For this review, take the finished solid that the model builds, in its own axes (mm). A direction names the side the tool comes from. Coordinates: 2 decimals unless noted, no trailing zeros. Loops run counter-clockwise (first coordinate to the right, second up) from the corner with the lowest first, then second, coordinate; pieces in that order, holes last. Notation, with made-up numbers: (-25.75, 40) -> (6.25, 40) arc R14 cw to (6.25, 61) -> close; hole circle Ø1 at (-10.5, 32). An arc over 180 degrees is marked (long way). One line per item, written item: value.
from build123d import *

# Parameters (mm, degrees)
SKETCH_1_W              = 200
SKETCH_1_H              = 213
EXTRUDE_1_DEPTH         = 4
EXTRUDE_2_DEPTH         = 54
CUT_EXTRUDE_2_DEPTH     = 298.880848663
CUT_EXTRUDE_3_DEPTH     = 42
SKETCH_7_R              = 1.8
SKETCH_7_R_2            = 11.5
CUT_EXTRUDE_4_DEPTH     = 282.53330176
MIRROR_START            = 176
MIRROR_1_OUTLINE_R      = 1.8
MIRROR_1_OUTLINE_R_2    = 11.5
MIRROR_1_DEPTH          = 3.5
CUT_EXTRUDE_START       = -21
CUT_EXTRUDE_5_OUTLINE_W = 27
CUT_EXTRUDE_5_OUTLINE_H = 20
CUT_EXTRUDE_5_DEPTH     = 21
CUT_EXTRUDE_START_2     = -6
CUT_EXTRUDE_6_OUTLINE_W = 27
CUT_EXTRUDE_6_OUTLINE_H = 28
CUT_EXTRUDE_6_DEPTH     = 6
CHAMFER_1_SIZE          = 4
CUT_EXTRUDE_START_3     = -54
CUT_EXTRUDE_7_DEPTH     = 54
EXTRUDE_3_DEPTH         = 10


# Read off the part's stored shape, not the designer's step: 镜向1, 切除-拉伸5, 切除-拉伸6
with BuildPart() as part:
    # 草图1 → 凸台-拉伸1 (new body)
    with BuildSketch(Plane(origin=(0, 0, 0), x_dir=(1, 0, 0), z_dir=(0, 1, 0))):
        with Locations((100, 106.5)):
            Rectangle(SKETCH_1_W, SKETCH_1_H)
    extrude(amount=EXTRUDE_1_DEPTH)

    # 草图1<4> → 凸台-拉伸2 (add)
    with BuildSketch(Plane(origin=(0, 0, 0), x_dir=(1, 0, 0), z_dir=(0, 1, 0))):
        with BuildLine():
            Line((0, 213), (0, 0))
            ThreePointArc((0, 0), (21.966991411, 53.033008589), (75, 75))
            Line((75, 75), (75, 213))
            Line((75, 213), (0, 213))
        make_face()
        with BuildLine():
            Line((125, 213), (125, 75))
            ThreePointArc((125, 75), (178.033008589, 53.033008589), (200, 0))
            Line((200, 0), (200, 213))
            Line((200, 213), (125, 213))
        make_face()
    extrude(amount=-EXTRUDE_2_DEPTH)

    # 草图3 → 切除-拉伸2 (cut, through all)
    with BuildSketch(Plane.XZ.offset(54)):
        Polygon((20.5, -186), (20.5, -165), (20.5, -144), (20.5, -117), (0, -117), (0, -213), (20.5, -213), align=None)
        Polygon((179.5, -117), (200, -117), (200, -213), (179.5, -213), (179.5, -165), align=None)
    extrude(amount=-CUT_EXTRUDE_2_DEPTH, mode=Mode.SUBTRACT)

    # 草图5 → 切除-拉伸3 (cut)
    with BuildSketch(Plane.XZ.offset(54)):
        Polygon((176, -165), (176, -144), (125, -144), (125, -186), (176, -186), align=None)
        Polygon((24, -165), (24, -144), (75, -144), (75, -186), (24, -186), align=None)
    extrude(amount=-CUT_EXTRUDE_3_DEPTH, mode=Mode.SUBTRACT)

    # 草图7 → 切除-拉伸4 (cut, through all)
    with BuildSketch(Plane(origin=(24, 0, 0), x_dir=(0, 0, -1), z_dir=(1, 0, 0))):
        with Locations((180.5, -17.5)):
            Circle(SKETCH_7_R)
        with Locations((149.5, -17.5)):
            Circle(SKETCH_7_R)
        with Locations((165, -33)):
            Circle(SKETCH_7_R_2)
        with Locations((180.5, -48.5)):
            Circle(SKETCH_7_R)
        with Locations((149.5, -48.5)):
            Circle(SKETCH_7_R)
    extrude(amount=-CUT_EXTRUDE_4_DEPTH, mode=Mode.SUBTRACT)

    # 镜向1 outline → 镜向1 (cut)
    with BuildSketch(Plane.YZ.offset(MIRROR_START)):
        with Locations((-17.5, -180.5)):
            Circle(MIRROR_1_OUTLINE_R)
        with Locations((-17.5, -149.5)):
            Circle(MIRROR_1_OUTLINE_R)
        with Locations((-33, -165)):
            Circle(MIRROR_1_OUTLINE_R_2)
        with Locations((-48.5, -180.5)):
            Circle(MIRROR_1_OUTLINE_R)
        with Locations((-48.5, -149.5)):
            Circle(MIRROR_1_OUTLINE_R)
    extrude(amount=MIRROR_1_DEPTH, mode=Mode.SUBTRACT)

    # 切除-拉伸5 outline → 切除-拉伸5 (cut)
    with BuildSketch(Plane(origin=(75, 0, 0), x_dir=(0, 0, -1), z_dir=(1, 0, 0)).offset(CUT_EXTRUDE_START)):
        with Locations((199.5, -33)):
            Rectangle(CUT_EXTRUDE_5_OUTLINE_W, CUT_EXTRUDE_5_OUTLINE_H)
    extrude(amount=CUT_EXTRUDE_5_DEPTH, mode=Mode.SUBTRACT)

    # 切除-拉伸6 outline → 切除-拉伸6 (cut)
    with BuildSketch(Plane.ZY.offset(-125).offset(CUT_EXTRUDE_START_2)):
        with Locations((-199.5, -33)):
            Rectangle(CUT_EXTRUDE_6_OUTLINE_W, CUT_EXTRUDE_6_OUTLINE_H)
    extrude(amount=CUT_EXTRUDE_6_DEPTH, mode=Mode.SUBTRACT)

    # 倒角1
    chamfer_1_edges = [part.edges().sort_by_distance(p)[0] for p in [
        (20.5, -25, -117),
        (179.5, -25, -117),
    ]]
    chamfer(chamfer_1_edges, length=CHAMFER_1_SIZE)

    # 草图11 → 切除-拉伸7 (cut)
    with BuildSketch(Plane.XZ.offset(54).offset(CUT_EXTRUDE_START_3)):
        with BuildLine():
            Line((75, -144), (10.975621098, -39.0625))
            ThreePointArc((10.975621098, -39.0625), (38.289562111, -65.401404801), (75, -75))
            Line((75, -75), (75, -144))
        make_face()
        with BuildLine():
            Line((125, -144), (125, -75))
            ThreePointArc((125, -75), (161.710437889, -65.401404801), (189.024378902, -39.0625))
            Line((189.024378902, -39.0625), (125, -144))
        make_face()
    extrude(amount=CUT_EXTRUDE_7_DEPTH, mode=Mode.SUBTRACT)

    # 草图12 → 凸台-拉伸3 (add)
    with BuildSketch(Plane(origin=(0, -54, 0), x_dir=(-1, 0, 0), z_dir=(0, -1, 0))):
        with BuildLine():
            Line((-9.993972793, 71.605361452), (-1.667158175, 86.766701767))
            ThreePointArc((-1.667158175, 86.766701767), (0, 93.265459675), (-1.667158175, 99.764217583))
            Line((-1.667158175, 99.764217583), (-9.993972793, 114.925557899))
            ThreePointArc((-9.993972793, 114.925557899), (-13.5, 117), (-17.006027207, 114.925557899))
            Line((-17.006027207, 114.925557899), (-25.332841825, 99.764217583))
            ThreePointArc((-25.332841825, 99.764217583), (-27, 93.265459675), (-25.332841825, 86.766701767))
            Line((-25.332841825, 86.766701767), (-17.006027207, 71.605361452))
            ThreePointArc((-17.006027207, 71.605361452), (-13.5, 69.53091935), (-9.993972793, 71.605361452))
        make_face()
        with BuildLine():
            Line((-190.006027207, 114.925557899), (-198.332841825, 99.764217583))
            ThreePointArc((-198.332841825, 99.764217583), (-200, 93.265459675), (-198.332841825, 86.766701767))
            Line((-198.332841825, 86.766701767), (-190.006027207, 71.605361452))
            ThreePointArc((-190.006027207, 71.605361452), (-186.5, 69.53091935), (-182.993972793, 71.605361452))
            Line((-182.993972793, 71.605361452), (-174.667158175, 86.766701767))
            ThreePointArc((-174.667158175, 86.766701767), (-173, 93.265459675), (-174.667158175, 99.764217583))
            Line((-174.667158175, 99.764217583), (-182.993972793, 114.925557899))
            ThreePointArc((-182.993972793, 114.925557899), (-186.5, 117), (-190.006027207, 114.925557899))
        make_face()
    extrude(amount=EXTRUDE_3_DEPTH)


solid = part.part
1. Insertion check: pin 1 Ø22.5 at (x, z) = (32.5, -56.5) entering from -Y; pin 2 Ø20.5 at (y, z) = (-33, -165) entering from +X; pin 3 Ø4.5 at (y, z) = (-17.5, -180.5) entering from -X; pin 4 Ø18.5 at (y, z) = (-17, -192) entering from +X. Each pin has a flat end and moves straight along its axis. Give the tip position at first contact, or say it passes through.
Return value:
pin 1: stops at y = -54
pin 2: passes through
pin 3: stops at x = 20.5
pin 4: stops at x = 179.5
2. For faces 5 (the flat face through (43.44, -26.62, -92.27)), 6 (the flat face through (4, -54, -110)), 7 (the flat face through (179.5, -19, -166)), 8 (the flat face through (178.772, -58.93, -107.239)), list the 3-axis set-ups (+Z, -Z, +X, -X, +Y, -Y) from which the entire face can be reached by the end or side of a thin tool; tool diameter is ignored.
Return value:
face 5: +Z, -Y
face 6: -Z, -X, -Y
face 7: -Z, +X, +Y, -Y
face 8: -Z, -Y
3. Take a section at D-D, the plane z = -84. Give the boundary of the cut face in (x, y), and give its area (3 significant figures).
Return value:
outline: (0, -54) -> (3.19, -54) -> (3.19, -64) -> (23.81, -64) -> (23.81, -54) -> (38.39, -54) -> (38.39, 0) -> (161.61, 0) -> (161.61, -54) -> (176.19, -54) -> (176.19, -64) -> (196.81, -64) -> (196.81, -54) -> (200, -54) -> (200, 4) -> (0, 4) -> close
area: 5,360 mm2
4. To check wall thickness, follow probe 1 along Y at (x, z) = (22.05, -180.5); probe 2 along Z at (x, y) = (178, -17); probe 3 along X at (y, z) = (-52, -172). State the ranges of each line that lie inside material, in increasing order. Write a range as from..to.
Return value:
probe 1: y = -54..-50.3, -46.7..-19.3, -15.7..4
probe 2: z = -213..-182.23, -178.77..-151.23, -147.77..-57.13
probe 3: x = 20.5..24, 176..179.5
5. Take a section at C-C, the plane x = 141. Give the boundary of the cut face in (y, z).
Return value:
outline: (-54, -213) -> (4, -213) -> (4, 0) -> (0, 0) -> (0, -117.78) -> (-54, -117.78) -> (-54, -144) -> (-12, -144) -> (-12, -186) -> (-54, -186) -> close
6. Take a section at B-B, the plane z = -165. Give the boundary of the cut face in (x, y).
Return value:
outline: (20.5, -54) -> (24, -54) -> (24, -44.5) -> (20.5, -44.5) -> close; (20.5, -21.5) -> (24, -21.5) -> (24, -12) -> (75, -12) -> (75, 0) -> (125, 0) -> (125, -12) -> (176, -12) -> (176, -21.5) -> (179.5, -21.5) -> (179.5, 4) -> (20.5, 4) -> close; (176, -54) -> (179.5, -54) -> (179.5, -44.5) -> (176, -44.5) -> close
7. The part is to be moulded in two halves that separate along Y. For faces 1 (the cylindrical face through (22.27, -32.49, -153.51)), 2 (the flat face through (128, -19, -200)), 3 (the flat face through (157.46, -26.62, -90.8)), 4 (the flat face through (99, 4, -108)), say which applies: pulls with the +Y half, pulls with the -Y half, needs draft (parallel to the pull), parting line crosses it, or undercut.
Return value:
face 1: undercut
face 2: undercut
face 3: needs draft
face 4: pulls with the +Y half
8. Take a section at A-A, the plane y = -33. Give the number of separate pieces and of enclosed holes in the cut face, and give its area (3 significant figures).
Return value:
separate pieces: 4
enclosed holes: 0
area: 10,600 mm2
